Could you check a few things on this model? Use its own coordinates, in mm. A direction names the side the tool comes from. Coordinates: 2 decimals unless noted, no trailing zeros. Order: outer loops, then holes, each group sorted by start corner. A loop starts at its lowest first (then second) coordinate and runs counter-clockwise, first axis right, second up. Notation, with made-up numbers: (-40, 59) - (-18, 59) arc R16 cw to (-18, 90) - close; hole circle Ø7 at (54, -1.75). An arc over 180 degrees is marked (long way). One line per item, written item: value.
from build123d import *

# Parameters (mm, degrees)
F0_W      = 285.75
F0_H      = 279.4
F1_DEPTH  = 3.175
F2_W      = 285.75
F2_H      = 66.675
F3_DEPTH  = 215.9
F4_W      = 58.7375
F4_H      = 100.0125
F5_DEPTH  = 285.75
F6_W      = 285.75
F6_H      = 4.7625
F7_DEPTH  = 279.4
F9_DEPTH  = 25.4
F10_W     = 63.5
F10_H     = 279.4
F10_W_2   = 7.9375
F11_DEPTH = 3.175
F12_W     = 63.5
F12_H     = 279.4
F12_W_2   = 7.9375
F13_DEPTH = 3.175
F14_W     = 69.85
F14_H     = 71.4375
F15_DEPTH = 101.6
F17_DEPTH = 71.4375
F18_W     = 69.85
F18_H     = 71.4375
F19_DEPTH = 101.6
F21_DEPTH = 71.4375
F24_W     = 292.1
F24_H     = 25.4
F25_DEPTH = 6.35
F22_W     = 71.4375
F22_H     = 114.3
F22_H_2   = 4.4173913043
F26_DEPTH = 3.175
F23_W     = 71.4375
F23_H     = 4.4173913043
F23_H_2   = 114.3
F27_DEPTH = 3.175
F29_DEPTH = 101.6
F31_DEPTH = 25.4
F33_DEPTH = 101.6
F35_DEPTH = 25.4


with BuildPart() as f1:
    # F0 (on Front) → F1 (new body)
    with BuildSketch(Plane.XZ):
        with Locations((142.875, 139.7)):
            Rectangle(F0_W, F0_H)
    extrude(amount=F1_DEPTH)

    # F2 (on face) → F3 (join)
    with BuildSketch(Plane.XY.offset(279.4)):
        with Locations((142.875, -33.3375)):
            Rectangle(F2_W, F2_H)
    extrude(amount=F3_DEPTH)

    # F4 (on face) → F5 (cut)
    with BuildSketch(Plane.YZ.offset(285.75)):
        with Locations((-37.30625, 329.40625)):
            Rectangle(F4_W, F4_H)
        with BuildLine():
            Line((-7.9375, 379.4125), (-7.9375, 438.15))
            ThreePointArc((-7.9375, 438.15), (-25.1413154401, 396.6163154401), (-66.675, 379.4125))
            Line((-66.675, 379.4125), (-7.9375, 379.4125))
        make_face()
        with BuildLine():
            Line((-7.9375, 438.15), (-66.675, 438.15))
            Line((-66.675, 438.15), (-66.675, 379.4125))
            ThreePointArc((-66.675, 379.4125), (-25.1413154401, 396.6163154401), (-7.9375, 438.15))
        make_face()
        with BuildLine():
            Line((-53.1113940543, 495.3), (-66.675, 495.3))
            Line((-66.675, 495.3), (-66.675, 438.15))
            Line((-66.675, 438.15), (-7.9375, 438.15))
            ThreePointArc((-7.9375, 438.15), (-20.5947102305, 474.5739042527), (-53.1113940543, 495.3))
        make_face()
    extrude(amount=-F5_DEPTH, mode=Mode.SUBTRACT)

    # F6 (on face) → F7 (join)
    with BuildSketch(Plane(origin=(0, 0, 279.4), x_dir=(1, 0, 0), z_dir=(0, 0, -1))):
        with Locations((142.875, 5.55625)):
            Rectangle(F6_W, F6_H)
    extrude(amount=F7_DEPTH)

    # F8 (on face) → F9 (cut)
    with BuildSketch(Plane(origin=(0, 0, 0), x_dir=(-1, 0, 0), z_dir=(0, 1, 0))):
        Polygon((-227.0125, 50.8), (-142.875, 50.8), (-58.7375, 50.8), (-58.7375, 219.075), (-227.0125, 219.075), align=None)
    extrude(amount=-F9_DEPTH, mode=Mode.SUBTRACT)

    # F10 (on face) → F11 (join)
    with BuildSketch(Plane.YZ.offset(285.75)):
        with Locations((-39.6875, 139.7)):
            Rectangle(F10_W, F10_H)
        with Locations((-3.96875, 139.7)):
            Rectangle(F10_W_2, F10_H)
    extrude(amount=F11_DEPTH)

    # F12 (on face) → F13 (join)
    with BuildSketch(Plane(origin=(0, 0, 0), x_dir=(0, -1, 0), z_dir=(-1, 0, 0))):
        with Locations((39.6875, 139.7)):
            Rectangle(F12_W, F12_H)
        with Locations((3.96875, 139.7)):
            Rectangle(F12_W_2, F12_H)
    extrude(amount=F13_DEPTH)

    # F14 (on face) → F15 (join)
    with BuildSketch(Plane.XY.offset(279.4)):
        Polygon((0, -7.9375), (0, 0), (-3.175, 0), (-3.175, -71.4375), (0, -71.4375), align=None)
        with Locations((-38.1, -35.71875)):
            Rectangle(F14_W, F14_H)
    extrude(amount=F15_DEPTH)

    # F16 (on face) → F17 (cut)
    with BuildSketch(Plane.XZ.offset(71.4375)):
        Polygon((-73.025, 279.4), (-3.175, 279.4), (-40.2302153021, 330.9550821594), (-73.025, 376.5826086957), align=None)
        Polygon((-38.1367188436, 332.4597827389), (0, 279.4), (0, 381), (-73.025, 381), align=None)
    extrude(amount=-F17_DEPTH, mode=Mode.SUBTRACT)

    # F18 (on face) → F19 (join)
    with BuildSketch(Plane.XY.offset(279.4)):
        Polygon((288.925, 0), (285.75, 0), (285.75, -7.9375), (285.75, -71.4375), (288.925, -71.4375), align=None)
        with Locations((323.85, -35.71875)):
            Rectangle(F18_W, F18_H)
    extrude(amount=F19_DEPTH)

    # F20 (on face) → F21 (cut)
    with BuildSketch(Plane.XZ.offset(71.4375)):
        Polygon((285.75, 381), (285.75, 279.4), (324.7502719302, 333.6612479029), (358.775, 381), align=None)
        Polygon((326.8437683887, 332.1565473234), (288.925, 279.4), (358.775, 279.4), (358.775, 376.5826086957), align=None)
    extrude(amount=-F21_DEPTH, mode=Mode.SUBTRACT)

    # F24 (on face) → F25 (join)
    with BuildSketch(Plane.XZ.offset(71.4375)):
        with Locations((142.875, 266.7)):
            Rectangle(F24_W, F24_H)
    extrude(amount=F25_DEPTH)

    # F22 (on face) → F26 (join)
    with BuildSketch(Plane.YZ.offset(358.775)):
        with Locations((-35.71875, 438.15)):
            Rectangle(F22_W, F22_H)
        with Locations((-35.71875, 378.7913043478)):
            Rectangle(F22_W, F22_H_2)
    extrude(amount=F26_DEPTH)

    # F23 (on face) → F27 (join)
    with BuildSketch(Plane(origin=(-73.025, 0, 0), x_dir=(0, -1, 0), z_dir=(-1, 0, 0))):
        with Locations((35.71875, 378.7913043478)):
            Rectangle(F23_W, F23_H)
        with Locations((35.71875, 438.15)):
            Rectangle(F23_W, F23_H_2)
    extrude(amount=F27_DEPTH)

    # F28 (on face) → F29 (join)
    with BuildSketch(Plane(origin=(0, 0, 0), x_dir=(0, -1, 0), z_dir=(-1, 0, 0))):
        Polygon((7.9375, 495.3), (0, 495.3), (0, 279.4), (7.9375, 279.4), (7.9375, 438.15), align=None)
    extrude(amount=F29_DEPTH)

    # F30 (on face) → F31 (cut)
    with BuildSketch(Plane.XZ.offset(7.9375)):
        Polygon((-76.2, 376.5826086957), (-76.2, 495.3), (-101.6, 495.3), (-101.6, 279.4), (-3.175, 279.4), (-73.025, 376.5826086957), align=None)
    extrude(amount=-F31_DEPTH, mode=Mode.SUBTRACT)

    # F32 (on face) → F33 (join)
    with BuildSketch(Plane.YZ.offset(285.75)):
        Polygon((0, 279.4), (0, 495.3), (-7.9375, 495.3), (-7.9375, 438.15), (-7.9375, 279.4), align=None)
    extrude(amount=F33_DEPTH)

    # F34 (on face) → F35 (cut)
    with BuildSketch(Plane.XZ.offset(7.9375)):
        Polygon((387.35, 495.3), (361.95, 495.3), (361.95, 376.5826086957), (358.775, 376.5826086957), (288.925, 279.4), (387.35, 279.4), align=None)
    extrude(amount=-F35_DEPTH, mode=Mode.SUBTRACT)


solid = f1.part
Item 1: Thinking about a two-plate mould opening in X: for faces 6 (the face through (324.34, -36.22, 328.67)), 7 (the face through (285.75, -39, 138)), 8 (the face through (144, -4, 0)), which applies, pulls with the +X half, pulls with the -X half, needs draft (parallel to the pull), parting line crosses it, or undercut?
Conclusion:
face 6: pulls with the +X half
face 7: undercut
face 8: needs draft
Item 2: For faces 1 (the face through (141, -77.788, 267)), 2 (the face through (-37.024, -40.132, 330.911)), 3 (the face through (288.925, -38, 138)), 4 (the face through (-3.175, -38, 138)), 5 (the face through (141, -71.438, 267)), which set-ups out of +Z, -Z, +X, -X, +Y, -Y let a thin tool reach every point of the face, with its end or its side?
Conclusion:
face 1: +Z, -Z, +X, -X, -Y
face 2: +Z, -Y
face 3: -Z, +X, +Y, -Y
face 4: -Z, -X, +Y, -Y
face 5: +Z, -Z
Item 3: If I drill on probe 1 along X at (y, z) = (-49.5, 423) (3 decimals); probe 2 along X at (y, z) = (-30, 147) (3 decimals); probe 3 along Y at (x, z) = (142, 375), over which ranges is the centre line in solid material (lowest first)?
Conclusion:
probe 1: -76.2 to -73.025, 358.775 to 361.95
probe 2: -3.175 to 0, 285.75 to 288.925
probe 3: -7.94 to 0
Item 4: I want a section at C-C on y = -65. Please give me the cut outline in (x, z) (3 decimals), then the cut area to 3 significant figures.
Conclusion:
outline: (-76.2, 376.583) - (-73.025, 376.583) - (-3.175, 279.4) - (-3.175, 0) - (0, 0) - (0, 279.4) - (-73.025, 381) - (-73.025, 495.3) - (-76.2, 495.3) - close; (285.75, 0) - (288.925, 0) - (288.925, 279.4) - (358.775, 376.583) - (361.95, 376.583) - (361.95, 495.3) - (358.775, 495.3) - (358.775, 381) - (285.75, 279.4) - close
area: 3,160 mm²
Item 5: I want a section at D-D on x = 220. Give the number of separate pieces and of enclosed holes in the cut face, then the cut area to 3 significant figures.
Conclusion:
separate pieces: 3
enclosed holes: 0
area: 3,420 mm²
Item 6: I'm going to push flat-ended pins straight in: pin 1 Ø6.5 at (y, z) = (-2.5, 148) entering from +X (3 decimals); pin 2 Ø5 at (x, y) = (107.5, -74.5) entering from +Z; pin 3 Ø1.5 at (x, z) = (10.5, 133) entering from -Y. Where does each tip first touch, or does it pass through?
Conclusion:
pin 1: x = 288.925
pin 2: z = 279.4
pin 3: y = -7.94
